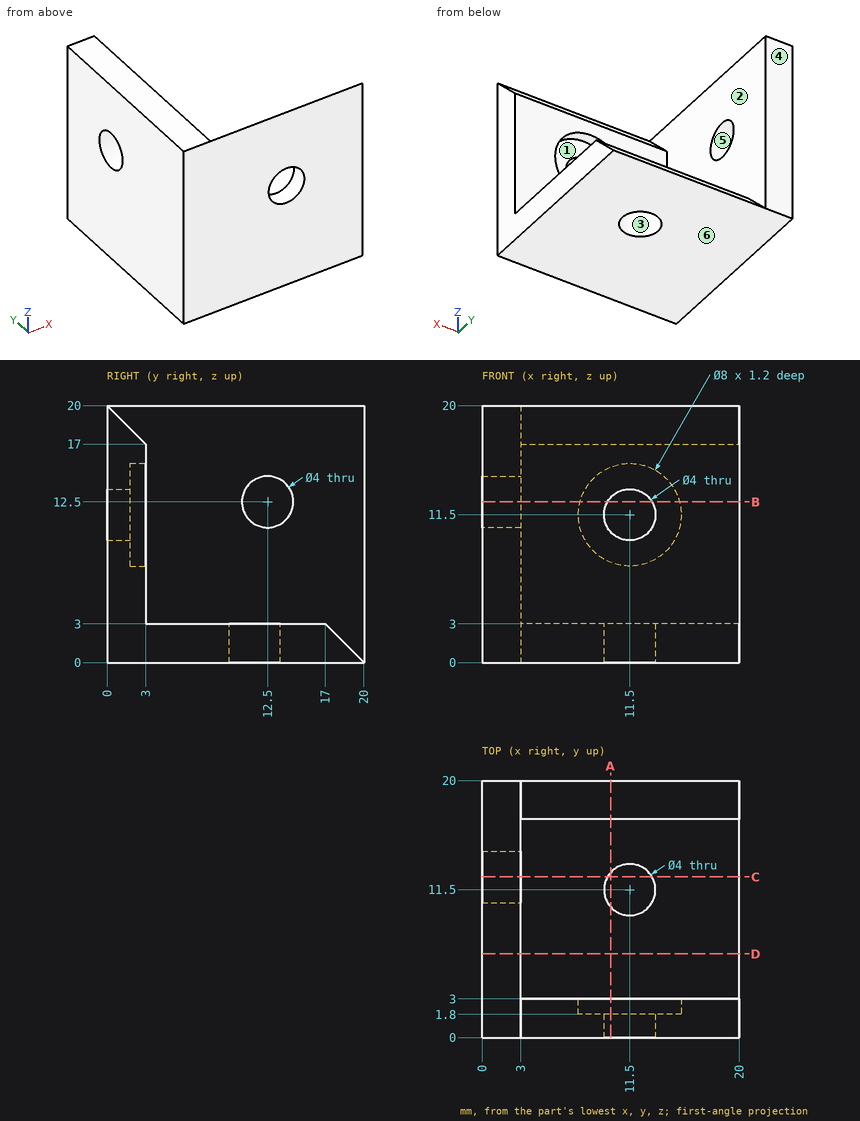
The figure shows three views and two pictorial views of one solid part (mm, origin at its lowest corner). Answer the questions. A direction names the side the tool comes from. Give positions to 0.01 mm unless a question says otherwise; leave off trailing zeros. Order: outer loops, then holes, each group sorted by start corner. A loop starts at its lowest first (then second) coordinate and runs counter-clockwise, first axis right, second up. Notation, with made-up numbers: (6, -34) -> (38, -34) arc R8 ccw to (38, -26) -> close; hole circle Ø4 at (6.25, 39). An arc over 180 degrees is marked (long way). Answer as CSV lines item,"result". Start each with the question number.
(1) Consider line 1 along Y through (x, z) = (2.1, 12.5); line 2 along Z through (x, y) = (18.5, 15.75). Determine where each line is inside the solid, lowest interval first.
(2) Section A-A, the plane x = 10 is taken. Write down the section's boundary in (y, z), plus the area to 3 significant figures.
(3) Which of the six approach directions +Z, -Z, +X, -X, +Y, -Y give full straight-line access (tool end or side, diameter ignored) to the marked faces 1, 2 and 3?
(4) For a pull along Z with two mould halves and no side action, classify the marked faces 4, 5 and 6 as released by +Z, released by -Z, zero draft, split by the parting line, or undercut.
(5) Section D-D, the plane y = 6.5 is taken. Write down the section's boundary in (x, z), plus the area to 3 significant figures.
(6) Section B-B, the plane z = 12.5 is taken. Write down the section's boundary in (x, y).
(7) Section C-C, the plane y = 12.5 is taken. Write down the section's boundary in (x, z), plus the area to 3 significant figures.
(8) Each of these flat-tipped pins is pushed along its axis until it touches: pin 1 Ø3 at (x, z) = (11, 11) entering from +Y; pin 2 Ø9 at (x, z) = (10, 11.5) entering from +Y; pin 3 Ø6 at (x, y) = (7.5, 12) entering from +Z. Where does it stop, or does it pass through?
Entries:
1,line 1,"0 to 10.5, 14.5 to 20"
1,line 2,"0 to 3"
2,outline,"(0, 0) -> (10.18, 0) -> (10.18, 3) -> (3, 3) -> (3, 7.79) -> (1.8, 7.79) -> (1.8, 10.18) -> (0, 10.18) -> close; (0, 12.82) -> (1.8, 12.82) -> (1.8, 15.21) -> (3, 15.21) -> (3, 17) -> (0, 20) -> close; (12.82, 0) -> (20, 0) -> (17, 3) -> (12.82, 3) -> close"
2,area,"80.4 mm²"
3,face 1,"+Y"
3,face 2,"+Z, +X, +Y"
3,face 3,"+Z, -Z"
4,face 4,"zero draft"
4,face 5,"undercut"
4,face 6,"released by -Z"
5,outline,"(0, 0) -> (20, 0) -> (20, 3) -> (3, 3) -> (3, 20) -> (0, 20) -> close"
5,area,"111 mm²"
6,outline,"(0, 0) -> (9.77, 0) -> (9.77, 1.8) -> (7.63, 1.8) -> (7.63, 3) -> (3, 3) -> (3, 10.5) -> (0, 10.5) -> close; (0, 14.5) -> (3, 14.5) -> (3, 20) -> (0, 20) -> close; (13.23, 0) -> (20, 0) -> (20, 3) -> (15.37, 3) -> (15.37, 1.8) -> (13.23, 1.8) -> close"
7,outline,"(0, 0) -> (9.77, 0) -> (9.77, 3) -> (3, 3) -> (3, 10.5) -> (0, 10.5) -> close; (0, 14.5) -> (3, 14.5) -> (3, 20) -> (0, 20) -> close; (13.23, 0) -> (20, 0) -> (20, 3) -> (13.23, 3) -> close"
7,area,"88.6 mm²"
8,pin 1,"y = 1.8"
8,pin 2,"y = 3"
8,pin 3,"z = 3"
